from build123d import *

# Parameters (mm, degrees)
F0_W     = 213.36
F0_H     = 335.28
F1_DEPTH = 304.8
F2_T     = -11.4554
F3_R     = 50.8
F4_DEPTH = 11.4554


with BuildPart() as f1:
    # F0 (on Front) → F1 (new body)
    with BuildSketch(Plane.XZ):
        Rectangle(F0_W, F0_H)
    extrude(amount=F1_DEPTH)

    # F2
    f2_openings = [f1.faces().sort_by_distance(p)[0] for p in [
        (106.68, -152.4, 0),
    ]]
    offset(amount=F2_T, openings=f2_openings)

    # F3 (on face) → F4 (cut, through all)
    with BuildSketch(Plane(origin=(0, 0, -167.64), x_dir=(1, 0, 0), z_dir=(0, 0, -1))):
        with Locations((-40.64, 152.4)):
            Circle(F3_R)
    extrude(amount=-F4_DEPTH, mode=Mode.SUBTRACT)


solid = f1.part
Design review of the part built by this model. Coordinates are the model's own, in mm. A direction names the side the tool comes from. Give positions to 0.01 mm unless a question says otherwise; leave off trailing zeros. Order: outer loops, then holes, each group sorted by start corner. A loop starts at its lowest first (then second) coordinate and runs counter-clockwise, first axis right, second up. Notation, with made-up numbers: (32, 25) - (78, 25) arc R16 cw to (78, 49) - close; hole circle Ø8 at (17, -11). An arc over 180 degrees is marked (long way). Write item = value, one per line. Start each with the question number.
Q1. Tool access review of faces 4 (the face through (-47.25, -202.77, -161.99)), 5 (the face through (106.68, -298, -13)), 6 (the face through (4, -150, 156.185)): name each direction out of +Z, -Z, +X, -X, +Y, -Y from which nothing blocks a thin tool from reaching the whole face with its end or side.
Q2. We need section A-A on y = -152.4. State the section outline as (x, z) points.
Q3. We need section C-C on x = 80.5. State the section outline as (y, z) points.
Q4. We need section D-D on y = -19. State the section outline as (x, z) points.
Q5. Mouldability with a two-part tool opening along Y and no side actions: class faces 1 (the face through (27, -150, -156.185)), 2 (the face through (-1, -304.8, 2)), 3 (the face through (-106.68, -150, -2)) as released by +Y, released by -Y, zero draft, split by the parting line, or undercut.
Q6. To check wall thickness, follow L1, parallel to Z at x = -90, y = -69; L2, parallel to Y at x = 33, z = 136; L3, parallel to X at y = -152, z = -160. State the ranges of each line that lie inside material, in increasing order. Write a range as from..to.
Q7. Clearance check with flat-ended pins moving along their axes: pin 1 Ø2 at (x, z) = (12.5, -52.5) entering from +Y; pin 2 Ø12 at (y, z) = (-173, -57) entering from +X. State where each tip first meets the part, or that it passes through.
Q8. We need section B-B on z = 131. State the section outline as (x, y) points.
Working result:
q1.face_4 = -Z
q1.face_5 = +Z, -Z, +X, +Y, -Y
q1.face_6 = +X
q2.outline = (-106.68, -167.64) - (-91.44, -167.64) - (-91.44, -156.18) - (-95.22, -156.18) - (-95.22, 156.18) - (106.68, 156.18) - (106.68, 167.64) - (-106.68, 167.64) - close; (10.16, -167.64) - (106.68, -167.64) - (106.68, -156.18) - (10.16, -156.18) - close
q3.outline = (-304.8, -167.64) - (0, -167.64) - (0, 167.64) - (-304.8, 167.64) - close; hole (-293.34, -156.18) - (-11.46, -156.18) - (-11.46, 156.18) - (-293.34, 156.18) - close
q4.outline = (-106.68, -167.64) - (106.68, -167.64) - (106.68, -156.18) - (-95.22, -156.18) - (-95.22, 156.18) - (106.68, 156.18) - (106.68, 167.64) - (-106.68, 167.64) - close
q5.face_1 = undercut
q5.face_2 = released by -Y
q5.face_3 = zero draft
q6.L1 = -167.64..-156.18, 156.18..167.64
q6.L2 = -304.8..-293.34, -11.46..0
q6.L3 = -106.68..-91.44, 10.16..106.68
q7.pin_1 = 0
q7.pin_2 = -95.22
q8.outline = (-106.68, -304.8) - (106.68, -304.8) - (106.68, -293.34) - (-95.22, -293.34) - (-95.22, -11.46) - (106.68, -11.46) - (106.68, 0) - (-106.68, 0) - close
